Autodesk Inventor part; units mm, degrees
ref_plane "YZ Plane" through (0, 0, 0) normal (1, 0, 0) x (0, 1, 0)
ref_plane "XZ Plane" through (0, 0, 0) normal (0, 1, 0) x (-1, 0, 0)
ref_plane "XY Plane" through (0, 0, 0) normal (0, 0, 1) x (1, 0, 0)
sketch "Эскиз1" plane through (0, 0, 0) normal (0, 0, 1) x (1, 0, 0)
  line L0 (0, -87.7141) -> (4, -87.7141)
  line L1 (4, -87.7141) -> (4, -82.7141)
  line L2 (4, -82.7141) -> (0, -82.7141)
  line L3 (0, -82.7141) -> (0, -87.7141)
  line L4 (4, -77.7141) -> (0, -77.7141)
  line L5 (0, -82.7141) -> (0, -77.7141)
  line L6 (0, -82.7141) -> (4, -82.7141)
  line L7 (4, -77.7141) -> (4, -82.7141)
  line L8 (4, -67.7141) -> (0, -67.7141)
  line L9 (0, -72.7141) -> (0, -67.7141)
  line L10 (0, -72.7141) -> (4, -72.7141)
  line L11 (4, -67.7141) -> (4, -72.7141)
  line L12 (4, -57.7141) -> (0, -57.7141)
  line L13 (0, -62.7141) -> (0, -57.7141)
  line L14 (0, -62.7141) -> (4, -62.7141)
  line L15 (4, -57.7141) -> (4, -62.7141)
  line L16 (4, -47.7141) -> (0, -47.7141)
  line L17 (0, -52.7141) -> (0, -47.7141)
  line L18 (0, -52.7141) -> (4, -52.7141)
  line L19 (4, -47.7141) -> (4, -52.7141)
  line L20 (4, -37.7141) -> (0, -37.7141)
  line L21 (0, -42.7141) -> (0, -37.7141)
  line L22 (0, -42.7141) -> (4, -42.7141)
  line L23 (4, -37.7141) -> (4, -42.7141)
  line L24 (4, -27.7141) -> (0, -27.7141)
  line L25 (0, -32.7141) -> (0, -27.7141)
  line L26 (0, -32.7141) -> (4, -32.7141)
  line L27 (4, -27.7141) -> (4, -32.7141)
  line L28 (4, -17.7141) -> (0, -17.7141)
  line L29 (0, -22.7141) -> (0, -17.7141)
  line L30 (0, -22.7141) -> (4, -22.7141)
  line L31 (4, -17.7141) -> (4, -22.7141)
  line L32 (4, -7.7141) -> (0, -7.7141)
  line L33 (0, -12.7141) -> (0, -7.7141)
  line L34 (0, -12.7141) -> (4, -12.7141)
  line L35 (4, -7.7141) -> (4, -12.7141)
  line L36 (0, -2.7141) -> (4, -2.7141)
  line L37 (4, 0) -> (4, -2.7141)
  line L38 (0, 0) -> (4, 0)
  line L39 (0, -2.7141) -> (0, 0)
  line L40 (-199, -2.7141) -> (-195, -2.7141)
  line L41 (-195, 0) -> (-195, -2.7141)
  line L42 (-199, 0) -> (-195, 0)
  line L43 (-199, -2.7141) -> (-199, 0)
  line L44 (-195, -7.7141) -> (-199, -7.7141)
  line L45 (-199, -12.7141) -> (-199, -7.7141)
  line L46 (-199, -12.7141) -> (-195, -12.7141)
  line L47 (-195, -7.7141) -> (-195, -12.7141)
  line L48 (-195, -17.7141) -> (-199, -17.7141)
  line L49 (-199, -22.7141) -> (-199, -17.7141)
  line L50 (-199, -22.7141) -> (-195, -22.7141)
  line L51 (-195, -17.7141) -> (-195, -22.7141)
  line L52 (-195, -27.7141) -> (-199, -27.7141)
  line L53 (-199, -32.7141) -> (-199, -27.7141)
  line L54 (-199, -32.7141) -> (-195, -32.7141)
  line L55 (-195, -27.7141) -> (-195, -32.7141)
  line L56 (-195, -77.7141) -> (-199, -77.7141)
  line L57 (-199, -82.7141) -> (-199, -77.7141)
  line L58 (-199, -82.7141) -> (-195, -82.7141)
  line L59 (-195, -77.7141) -> (-195, -82.7141)
  line L60 (-195, -67.7141) -> (-199, -67.7141)
  line L61 (-199, -72.7141) -> (-199, -67.7141)
  line L62 (-199, -72.7141) -> (-195, -72.7141)
  line L63 (-195, -67.7141) -> (-195, -72.7141)
  line L64 (-195, -57.7141) -> (-199, -57.7141)
  line L65 (-199, -62.7141) -> (-199, -57.7141)
  line L66 (-199, -62.7141) -> (-195, -62.7141)
  line L67 (-195, -57.7141) -> (-195, -62.7141)
  line L68 (-199, -52.7141) -> (-199, -47.7141)
  line L69 (-195, -47.7141) -> (-199, -47.7141)
  line L70 (-199, -52.7141) -> (-199, -47.7141)
  line L71 (-199, -52.7141) -> (-195, -52.7141)
  line L72 (-195, -47.7141) -> (-195, -52.7141)
  line L73 (-195, -37.7141) -> (-199, -37.7141)
  line L74 (-199, -42.7141) -> (-199, -37.7141)
  line L75 (-199, -42.7141) -> (-195, -42.7141)
  line L76 (-195, -37.7141) -> (-195, -42.7141)
  line L77 (-195, -82.7141) -> (-199, -82.7141)
  line L78 (-199, -82.7141) -> (-199, -87.7141)
  line L79 (-199, -87.7141) -> (-195, -87.7141)
  line L80 (-195, -87.7141) -> (-195, -82.7141)
  line L81 (-195, 0) -> (0, 0)
  line L82 (0, 0) -> (0, -87.7141)
  line L83 (0, -87.7141) -> (-195, -87.7141)
  line L84 (-195, -87.7141) -> (-195, 0)
extrude "Выдавливание1" add sketch "Эскиз1" along normal blind 4 contours L83 L80 L59 L84 L63 L67 L72 L76 L55 L51 L47 L41 L81 L39 L82 L33 L29 L25 L21 L17 L13 L9 L5 L3 | L5 L4 L7 L2 | L58 L57 L56 L59 | L9 L8 L11 L10 | L62 L61 L60 L63 | L13 L12 L15 L14 | L66 L65 L64 L67 | L17 L16 L19 L18 | L71 L68 L69 L72 | L21 L20 L23 L22 | L75 L74 L73 L76 | L25 L24 L27 L26 | L54 L53 L52 L55 | L29 L28 L31 L30 | L50 L49 L48 L51 | L33 L32 L35 L34 | L46 L45 L44 L47 | L39 L38 L37 L36 | L40 L43 L42 L41
properties part number "KB33-046-004-017 - Крышка наклонная"
Source: CAD feature listing. Evaluate the final solid. Frame: model axes, mm. A direction names the side the tool comes from. Give positions to 0.01 mm unless a question says otherwise; leave off trailing zeros. Write each loop counter-clockwise with the first axis right and the second up, starting at its lowest first coordinate (ties: lowest second). Pieces come first, ordered by that corner, then holes. Notation, with made-up numbers: (85.5, -18) -> (136.5, -18) arc R31 cw to (136.5, 16) -> close; hole circle Ø8 at (15.5, -40). An arc over 180 degrees is marked (long way). Return JSON: item names as keys, results as strings. Group by question number.
1. Pin query (flat end, axial travel): pin 1 Ø1.2 at (y, z) = (-25, 2.5) entering from +X; pin 2 Ø1.2 at (x, z) = (-196.5, 2.5) entering from +Y; pin 3 Ø2 at (x, z) = (1.5, 1.5) entering from -Y. Return the tip coordinate at first contact, or that it passes through.
2. Access query for faces 1 (the face through (-195, -45, 2)), 2 (the face through (-195, -85, 2)), 3 (the face through (0, -15, 2)). Directions: +Z, -Z, +X, -X, +Y, -Y. A direction counts if a zero-diameter tool reaches every point of the face in a straight line with its end or side. Return the directions, or none.
3. Mould query, pull axis Y, two halves, no side actions, for faces 4 (the face through (4, -80, 2)), 5 (the face through (-197, -17.714, 2)). Classes: +Y half, -Y half, draft (parallel to the pull), parting line (faces both ways), or undercut.
4. Section A-A, the plane y = -44.5. Output: boundary loops of the cut face in (x, z), then the cut area to 3 significant figures.
5. Material intervals for line 1 (X direction, y = -45, z = 2.8), sorted ascending. Write a range as from..to.
Determined:
{
 "1": {"pin 1": "stops at x = 0", "pin 2": "stops at y = 0", "pin 3": "stops at y = -82.71"},
 "2": {"face 1": "+Z, -Z, -X", "face 2": "+Z, -Z, -X, -Y", "face 3": "+Z, -Z, +X"},
 "3": {"face 4": "draft", "face 5": "undercut"},
 "4": {"outline": "(-195, 0) -> (0, 0) -> (0, 4) -> (-195, 4) -> close", "area": "780 mm2"},
 "5": {"line 1": "x = -195..0"}
}
